Geometry: final body of the model. Coordinates: model frame, mm. A direction names the side the tool comes from. Round coordinates to 2 decimals unless told otherwise and drop trailing zeros. Order: outer loops, then holes, each group sorted by start corner. A loop starts at its lowest first (then second) coordinate and runs counter-clockwise, first axis right, second up. Notation, with made-up numbers: M 8,80.25 L 51,80.25 A29 cw 51,108.25 Z; hole C 8,-17.75 d10. An arc over 180 degrees is marked long. Put each result on its own line as item: value. Start each with the question number.
1) First-contact query: P1, Ø4, axis at y = -1, z = 0.5, coming from the +X side; P2, Ø6, axis at x = -1.5, y = 6.5, coming from the -Z side; P3, Ø6, axis at x = 8.5, z = 0.5, coming from the -Y side. Flat tips, straight axial feed; report the tip coordinate or a pass-through.
2) Draft query along X for faces 1 (the cylindrical face through (0, -14, -2)), 2 (the flat face through (-2.5, 0, 0)), 3 (the conical face through (-0.845, -22.625, 3.803)). Return one class per face: pulls with the +X half, pulls with the -X half, needs draft (parallel to the pull), parting line crosses it, or undercut.
3) Section A-A, the plane x = 0. Return loops of the section in (y, z).
4) Material intervals for probe 1 along Z at (x, y) = (0, -12.5); probe 2 along Z at (x, y) = (-3, 3.5), sorted ascending. Write a range as [from, to].
5) Section D-D, the plane x = 9.75. Return loops of the section in (y, z), then the cut area to 3 significant figures.
6) Section C-C, the plane y = 0. Return loops of the section in (x, z).
7) Access query for faces 4 (the cylindrical face through (4.344, 3.373, -2.15)), 5 (the flat face through (-4, 0, 0)), 6 (the flat face through (2, 25, 2)), 7 (the cylindrical face through (3.34, -11.18, -1.05)). Directions: +Z, -Z, +X, -X, +Y, -Y. A direction counts if a zero-diameter tool reaches every point of the face in a straight line with its end or side. Return the directions, or none.
8) Section B-B, the plane z = 0. Count the separate pieces of the cut face and the enclosed holes in it, then the cut area to 3 significant figures.
from build123d import *

# Parameters (mm, degrees)
SKETCH3_W           = 2.5
SKETCH3_H           = 25
SKETCH3_H_2         = 6.220476857
SKETCH3_H_3         = 18.779523143
BOSS_EXTRUDE2_START = 3.5
SKETCH5_R           = 5
BOSS_EXTRUDE2_DEPTH = 7.5
SKETCH6_R           = 4
CUT_EXTRUDE1_DEPTH  = 13.5
SKETCH7_R           = 2
CUT_EXTRUDE2_DEPTH  = 50


with BuildPart() as part:
    # Sketch3 → Revolve1 (revolve)
    with BuildSketch(Plane.XY):
        Polygon((2.5, 6.220476857), (2.5, 0), (3.5, 0), (3.5, 19), (4.5, 19), (3.5, 25), (2.5, 25), align=None)
        Polygon((2.5, 0), (2.5, -25), (3.5, -25), (4.5, -19), (3.5, -19), (3.5, 0), align=None)
        with Locations((1.25, -12.5)):
            Rectangle(SKETCH3_W, SKETCH3_H)
        with Locations((1.25, 3.110238429)):
            Rectangle(SKETCH3_W, SKETCH3_H_2)
        with Locations((1.25, 15.610238429)):
            Rectangle(SKETCH3_W, SKETCH3_H_3)
    revolve(axis=Axis((0, 0, 0), (0, 1, 0)))

    # Sketch5 → Boss-Extrude2 (add, symmetric)
    with BuildSketch(Plane(origin=(0, 0, 0), x_dir=(0, 0, -1), z_dir=(1, 0, 0)).offset(BOSS_EXTRUDE2_START)):
        Circle(SKETCH5_R)
    extrude(amount=BOSS_EXTRUDE2_DEPTH, both=True)

    # Sketch6 → Cut-Extrude1 (cut)
    with BuildSketch(Plane(origin=(11, 0, 0), x_dir=(0, 0, -1), z_dir=(1, 0, 0))):
        Circle(SKETCH6_R)
    extrude(amount=-CUT_EXTRUDE1_DEPTH, mode=Mode.SUBTRACT)

    # Sketch7 → Cut-Extrude2 (cut)
    with BuildSketch(Plane.XZ.offset(25)):
        Circle(SKETCH7_R)
    extrude(amount=-CUT_EXTRUDE2_DEPTH, mode=Mode.SUBTRACT)


solid = part.part
Result sheet:
1. P1: stops at x = -2.5
1. P2: stops at z = -3.57
1. P3: stops at y = -5
2. face 1: undercut
2. face 2: pulls with the +X half
2. face 3: parting line crosses it
3. outline: M -25,-3.5 L -19,-4.5 L -19,-3.5 L -3.57,-3.5 A5 ccw 3.57,-3.5 L 19,-3.5 L 19,-4.5 L 25,-3.5 L 25,-2 L 3.46,-2 A4 cw -3.46,-2 L -25,-2 Z; M -25,2 L -3.46,2 A4 cw 3.46,2 L 25,2 L 25,3.5 L 19,4.5 L 19,3.5 L 3.57,3.5 A5 ccw -3.57,3.5 L -19,3.5 L -19,4.5 L -25,3.5 Z
4. probe 1: z = [-3.5, -2], [2, 3.5]
4. probe 2: z = [-3.57, 3.57]
5. outline: C 0,0 d10; hole C 0,0 d8
5. area: 28.3 mm2
6. outline: M -4,-5 L 11,-5 L 11,-4 L -2.5,-4 L -2.5,4 L 11,4 L 11,5 L -4,5 Z
7. face 4: +X
7. face 5: +Z, -Z, -X
7. face 6: +Z, -Z, +X, -X, +Y
7. face 7: none
8. separate pieces: 3
8. enclosed holes: 0
8. area: 166 mm2
